```python
from build123d import *

# Parameters (mm, degrees)
SKETCH2_W           = 155
SKETCH2_H           = 105
BOSS_EXTRUDE1_DEPTH = 14
SKETCH3_R           = 53.5
CUT_EXTRUDE1_DEPTH  = 4
SKETCH4_R           = 32
CUT_EXTRUDE2_DEPTH  = 10
FILLET1_R           = 10
SKETCH5_R           = 2.25
CUT_EXTRUDE3_DEPTH  = 95.649352877
CUT_EXTRUDE4_DEPTH  = 95.649352877
SKETCH8_R           = 5
CUT_EXTRUDE6_DEPTH  = 2.5


with BuildPart() as part:
    # Sketch2 → Boss-Extrude1 (new body)
    with BuildSketch(Plane.XY):
        Rectangle(SKETCH2_W, SKETCH2_H)
    extrude(amount=BOSS_EXTRUDE1_DEPTH)

    # Sketch3 → Cut-Extrude1 (cut)
    with BuildSketch(Plane(origin=(0, 0, 0), x_dir=(-1, 0, 0), z_dir=(0, 0, -1))):
        with Locations((0, -0.5)):
            Circle(SKETCH3_R)
    extrude(amount=-CUT_EXTRUDE1_DEPTH, mode=Mode.SUBTRACT)

    # Sketch4 → Cut-Extrude2 (cut)
    with BuildSketch(Plane(origin=(0, 0, 4), x_dir=(-1, 0, 0), z_dir=(0, 0, -1))):
        with Locations((0, -0.5)):
            Circle(SKETCH4_R)
    extrude(amount=-CUT_EXTRUDE2_DEPTH, mode=Mode.SUBTRACT)

    # Fillet1
    fillet1_edges = [part.edges().sort_by_distance(p)[0] for p in [
        (77.5, -52.5, 7),
        (-77.5, -52.5, 7),
        (-77.5, 52.5, 7),
        (77.5, 52.5, 7),
    ]]
    fillet(fillet1_edges, radius=FILLET1_R)

    # Sketch5 → Cut-Extrude3 (cut, through all)
    with BuildSketch(Plane.XY.offset(14)):
        with Locations((43.884277794, 17.677463037)):
            Circle(SKETCH5_R)
        with Locations((43.884277794, -18.677463037)):
            Circle(SKETCH5_R)
        with Locations((-43.884277794, -18.677463037)):
            Circle(SKETCH5_R)
        with Locations((-43.884277794, 17.677463037)):
            Circle(SKETCH5_R)
    extrude(amount=-CUT_EXTRUDE3_DEPTH, mode=Mode.SUBTRACT)

    # Sketch6 → Cut-Extrude4 (cut, through all)
    with BuildSketch(Plane(origin=(0, 0, 0), x_dir=(-1, 0, 0), z_dir=(0, 0, -1))):
        with BuildLine():
            ThreePointArc((45.846474332, -4.255102041), (46, -0.5), (45.846474332, 3.255102041))
            ThreePointArc((45.846474332, 3.255102041), (48.591563829, 6.489987456), (51.826449245, 3.744897959))
            ThreePointArc((51.826449245, 3.744897959), (52, -0.5), (51.826449245, -4.744897959))
            ThreePointArc((51.826449245, -4.744897959), (48.591563829, -7.489987456), (45.846474332, -4.255102041))
        make_face()
    extrude(amount=-CUT_EXTRUDE4_DEPTH, mode=Mode.SUBTRACT)

    # Sketch8 → Cut-Extrude6 (cut)
    with BuildSketch(Plane(origin=(0, 0, 4), x_dir=(-1, 0, 0), z_dir=(0, 0, -1))):
        with Locations((43.884277794, 17.677463037)):
            Circle(SKETCH8_R)
        with Locations((43.884277794, -18.677463037)):
            Circle(SKETCH8_R)
        with Locations((-43.884277794, 17.677463037)):
            Circle(SKETCH8_R)
        with Locations((-43.884277794, -18.677463037)):
            Circle(SKETCH8_R)
    extrude(amount=-CUT_EXTRUDE6_DEPTH, mode=Mode.SUBTRACT)


solid = part.part
```
CAD build for the part. Positions are in the model's coordinates, mm. A direction names the side the tool comes from. Round coordinates to 2 decimals unless told otherwise and drop trailing zeros. Order: outer loops, then holes, each group sorted by start corner. A loop starts at its lowest first (then second) coordinate and runs counter-clockwise, first axis right, second up. Notation, with made-up numbers: (-38, 48.5) - (9, 48.5) arc R19 cw to (9, 81.5) - close; hole circle Ø1 at (-7, 10.25). An arc over 180 degrees is marked (long way). Use CSV: the item, a comma, the result in double quotes. Start each with the question number.
1) Saw through at C-C (z = 12.25). List the corners of the cut face in (x, y), and give its area (3 significant figures).
2) Pin check, flat tips, straight feed: pin 1 Ø6 at (x, y) = (-43.88, 17.68) entering from +Z; pin 2 Ø3 at (x, y) = (46.5, 17) entering from -Z; pin 3 Ø2.5 at (x, y) = (43.88, -18.68) entering from +Z; pin 4 Ø8 at (x, y) = (42, -17.5) entering from -Z. Stop position of each tip, or through.
3) Saw through at B-B (y = -0.5). List the corners of the cut face in (x, z).
4) Two-plate mould, pull along Y, no slides. Class faces 4 (the flat face through (-58, 1, 0)), 5 (the flat face through (-45, -21, 6.5)), 6 (the cylindrical face through (48.88, 17.9, 5.23)), 7 (the flat face through (-1, 52.5, 7)): pulls with the +Y half, pulls with the -Y half, needs draft (parallel to the pull), parting line crosses it, or undercut.
5) Tool access for faces 1 (the cylindrical face through (-52, -0.4, 8.9)), 2 (the flat face through (-77.5, -1, 7)), 3 (the cylindrical face through (47.57, -15.3, 5.23)): list every direction of +Z, -Z, +X, -X, +Y, -Y with a clear straight run to the whole face (end or side of a thin tool).
6) Saw through at D-D (x = -17). List the corners of the cut face in (y, z).
7) Wall check: L1, parallel to Y at x = -44, z = 13.25; L2, parallel to Y at x = -49, z = 12.75; L3, parallel to Y at x = 0, z = 11. Give the ranges that are in metal, low to high. Write a range as [from, to].
8) Saw through at A-A (x = 0). List the corners of the cut face in (y, z), and give its area (3 significant figures).
Values follow:
1,outline,"(-77.5, -42.5) arc R10 ccw to (-67.5, -52.5) - (67.5, -52.5) arc R10 ccw to (77.5, -42.5) - (77.5, 42.5) arc R10 ccw to (67.5, 52.5) - (-67.5, 52.5) arc R10 ccw to (-77.5, 42.5) - close; hole (-51.83, -4.74) arc R3 ccw to (-45.85, -4.26) arc R46 cw to (-45.85, 3.26) arc R3 ccw to (-51.83, 3.74) arc R52 ccw to start; hole circle Ø4.5 at (-43.88, -18.68); hole circle Ø4.5 at (-43.88, 17.68); hole circle Ø64 at (0, -0.5); hole circle Ø4.5 at (43.88, -18.68); hole circle Ø4.5 at (43.88, 17.68)"
1,area,"12,800 mm2"
2,pin 1,"stops at z = 14"
2,pin 2,"stops at z = 6.5"
2,pin 3,"passes through"
2,pin 4,"stops at z = 4"
3,outline,"(-77.5, 0) - (-53.5, 0) - (-53.5, 4) - (-52, 4) - (-52, 14) - (-77.5, 14) - close; (-46, 4) - (-32, 4) - (-32, 14) - (-46, 14) - close; (32, 4) - (53.5, 4) - (53.5, 0) - (77.5, 0) - (77.5, 14) - (32, 14) - close"
4,face 4,"needs draft"
4,face 5,"undercut"
4,face 6,"undercut"
4,face 7,"pulls with the +Y half"
5,face 1,"+Z, -Z"
5,face 2,"+Z, -Z, -X, +Y, -Y"
5,face 3,"-Z"
6,outline,"(-52.5, 0) - (-51.23, 0) - (-51.23, 4) - (-27.61, 4) - (-27.61, 14) - (-52.5, 14) - close; (26.61, 4) - (50.23, 4) - (50.23, 0) - (52.5, 0) - (52.5, 14) - (26.61, 14) - close"
7,L1,"y = [-52.5, -20.92], [-16.43, 15.43], [19.92, 52.5]"
7,L2,"y = [-52.5, -7.5], [6.5, 52.5]"
7,L3,"y = [-52.5, -32.5], [31.5, 52.5]"
8,outline,"(-52.5, 4) - (-32.5, 4) - (-32.5, 14) - (-52.5, 14) - close; (31.5, 4) - (52.5, 4) - (52.5, 14) - (31.5, 14) - close"
8,area,"410 mm2"
